```python
from build123d import *

# Parameters (mm, degrees)
F1_DEPTH = 10
F2_DEPTH = 12
F3_SIZE  = 5
F4_SIZE  = 1.99999
F5_R     = 10
F6_DEPTH = 5
F7_R     = 4.99999
F9_DEPTH = 9


# Not quite as in the source:
# - a fillet or chamfer is up to 0.001 mm smaller than in the source, because OpenCascade refuses the exact size


with BuildPart() as f1:
    # F0 (on Right) → F1 (new body)
    with BuildSketch(Plane.YZ):
        with BuildLine():
            Line((15, 5), (27.0370116692, 13))
            ThreePointArc((27.0370116692, 13), (21.2132034356, 21.2132034356), (13, 27.0370116692))
            Line((13, 27.0370116692), (5, 15))
            Line((5, 15), (0, 15))
            Line((0, 15), (-5, 15))
            Line((-5, 15), (-13, 27.0370116692))
            ThreePointArc((-13, 27.0370116692), (-21.2132034356, 21.2132034356), (-27.0370116692, 13))
            Line((-27.0370116692, 13), (-15, 5))
            Line((-15, 5), (-15, 0))
            Line((-15, 0), (-15, -5))
            Line((-15, -5), (-27.0370116692, -13))
            ThreePointArc((-27.0370116692, -13), (-21.2132034356, -21.2132034356), (-13, -27.0370116692))
            Line((-13, -27.0370116692), (-5, -15))
            Line((-5, -15), (0, -15))
            Line((0, -15), (5, -15))
            Line((5, -15), (13, -27.0370116692))
            ThreePointArc((13, -27.0370116692), (21.2132034356, -21.2132034356), (27.0370116692, -13))
            Line((27.0370116692, -13), (15, -5))
            Line((15, -5), (15, 0))
            Line((15, 0), (15, 5))
        make_face()
    extrude(amount=F1_DEPTH)

    # F0 (on Right) → F2 (join)
    with BuildSketch(Plane.YZ):
        with BuildLine():
            ThreePointArc((27.0370116692, -13), (29.2498747867, -6.6666952054), (30, 0))
            ThreePointArc((30, 0), (29.2498747867, 6.6666952054), (27.0370116692, 13))
            Line((27.0370116692, 13), (15, 5))
            Line((15, 5), (15, 0))
            Line((15, 0), (15, -5))
            Line((15, -5), (27.0370116692, -13))
        make_face()
        with BuildLine():
            ThreePointArc((27.0370116692, 13), (29.2498747867, 6.6666952054), (30, 0))
            ThreePointArc((30, 0), (29.2498747867, -6.6666952054), (27.0370116692, -13))
            Line((27.0370116692, -13), (34, -8))
            Line((34, -8), (34, 0))
            Line((34, 0), (34, 8))
            Line((34, 8), (27.0370116692, 13))
        make_face()
        with BuildLine():
            Line((5, 15), (13, 27.0370116692))
            ThreePointArc((13, 27.0370116692), (0, 30), (-13, 27.0370116692))
            Line((-13, 27.0370116692), (-5, 15))
            Line((-5, 15), (0, 15))
            Line((0, 15), (5, 15))
        make_face()
        with BuildLine():
            ThreePointArc((-13, 27.0370116692), (0, 30), (13, 27.0370116692))
            Line((13, 27.0370116692), (8, 34))
            Line((8, 34), (0, 34))
            Line((0, 34), (-8, 34))
            Line((-8, 34), (-13, 27.0370116692))
        make_face()
        with BuildLine():
            Line((-15, 5), (-27.0370116692, 13))
            ThreePointArc((-27.0370116692, 13), (-30, 0), (-27.0370116692, -13))
            Line((-27.0370116692, -13), (-15, -5))
            Line((-15, -5), (-15, 0))
            Line((-15, 0), (-15, 5))
        make_face()
        with BuildLine():
            ThreePointArc((-27.0370116692, -13), (-30, 0), (-27.0370116692, 13))
            Line((-27.0370116692, 13), (-34, 8))
            Line((-34, 8), (-34, 0))
            Line((-34, 0), (-34, -8))
            Line((-34, -8), (-27.0370116692, -13))
        make_face()
        with BuildLine():
            ThreePointArc((-13, -27.0370116692), (0, -30), (13, -27.0370116692))
            Line((13, -27.0370116692), (5, -15))
            Line((5, -15), (0, -15))
            Line((0, -15), (-5, -15))
            Line((-5, -15), (-13, -27.0370116692))
        make_face()
        with BuildLine():
            Line((8, -34), (13, -27.0370116692))
            ThreePointArc((13, -27.0370116692), (0, -30), (-13, -27.0370116692))
            Line((-13, -27.0370116692), (-8, -34))
            Line((-8, -34), (0, -34))
            Line((0, -34), (8, -34))
        make_face()
    extrude(amount=F2_DEPTH)

    # F3
    f3_edges = [f1.edges().sort_by_distance(p)[0] for p in [
        (10, 21.213203, 21.213203),
        (10, -21.213203, 21.213203),
        (10, -21.213203, -21.213203),
        (10, 21.213203, -21.213203),
    ]]
    chamfer(f3_edges, length=F3_SIZE)

    # F4 (size 2 in the source; OpenCascade refuses exactly that, so slightly less here)
    f4_edges = [f1.edges().sort_by_distance(p)[0] for p in [
        (12, 0, 34),
        (12, -10.5, 30.518506),
        (12, 10.5, 30.518506),
        (12, -9, 21.018506),
        (12, 9, 21.018506),
        (12, 0, 15),
        (12, -15, 0),
        (12, -21.018506, 9),
        (12, -30.518506, 10.5),
        (12, -34, 0),
        (12, -30.518506, -10.5),
        (12, -21.018506, -9),
        (12, 0, -15),
        (12, -9, -21.018506),
        (12, -10.5, -30.518506),
        (12, 0, -34),
        (12, 10.5, -30.518506),
        (12, 9, -21.018506),
        (12, 15, 0),
        (12, 21.018506, 9),
        (12, 30.518506, 10.5),
        (12, 34, 0),
        (12, 21.018506, -9),
        (12, 30.518506, -10.5),
    ]]
    chamfer(f4_edges, length=F4_SIZE)

    # F5 (on face) → F6 (join)
    with BuildSketch(Plane.YZ.offset(10)):
        Circle(F5_R)
    extrude(amount=F6_DEPTH)

    # F7 (radius 5 in the source; OpenCascade refuses exactly that, so slightly less here)
    f7_edges = [f1.edges().sort_by_distance(p)[0] for p in [
        (15, -10, 0),
    ]]
    fillet(f7_edges, radius=F7_R)

    # F8 (on face) → F9 (join)
    with BuildSketch(Plane.YZ):
        with BuildLine():
            ThreePointArc((0, -15), (10.6066017178, -10.6066017178), (15, 0))
            ThreePointArc((15, 0), (10.6066017178, 10.6066017178), (0, 15))
            ThreePointArc((0, 15), (-10.6066017178, 10.6066017178), (-15, 0))
            ThreePointArc((-15, 0), (-10.6066017178, -10.6066017178), (0, -15))
        make_face()
    extrude(amount=-F9_DEPTH)


solid = f1.part
```
Could you check a few things on this model? Use its own coordinates, in mm. A direction names the side the tool comes from. Give positions to 0.01 mm unless a question says otherwise; leave off trailing zeros. Write each loop counter-clockwise with the first axis right and the second up, starting at its lowest first coordinate (ties: lowest second). Pieces come first, ordered by that corner, then holes. Notation, with made-up numbers: (-31.75, 57.25) -> (-12.75, 57.25) arc R30 ccw to (-12.75, 89.25) -> close; hole circle Ø10 at (64, 24.25). An arc over 180 degrees is marked (long way). Write each question's results on one line, items separated by ' | '.
1. I want a section at B-B, the plane x = 1.75. Write out the boundary of the cut face in (y, z).
Check sheet entries:
outline: (-34, -8) -> (-27.04, -13) arc R30 ccw to (-13, -27.04) -> (-8, -34) -> (8, -34) -> (13, -27.04) arc R30 ccw to (27.04, -13) -> (34, -8) -> (34, 8) -> (27.04, 13) arc R30 ccw to (13, 27.04) -> (8, 34) -> (-8, 34) -> (-13, 27.04) arc R30 ccw to (-27.04, 13) -> (-34, 8) -> close
2. I need wall thicknesses on L1, parallel to X at y = 26, z = 2; L2, parallel to X at y = 9, z = 0.5; L3, parallel to Y at x = 14, z = -1.5. Which ranges of each line are inside material? Lowest first, please.
Check sheet entries:
L1: x = 0 to 12 | L2: x = -9 to 12.98 | L3: y = -7.86 to 7.86
3. I want a section at D-D, the plane x = 7.5. Write out the boundary of the cut face in (y, z).
Check sheet entries:
outline: (-34, -8) -> (-27.04, -13) -> (-24.93, -11.6) arc R27.5 ccw to (-11.6, -24.93) -> (-13, -27.04) -> (-8, -34) -> (8, -34) -> (13, -27.04) -> (11.6, -24.93) arc R27.5 ccw to (24.93, -11.6) -> (27.04, -13) -> (34, -8) -> (34, 8) -> (27.04, 13) -> (24.93, 11.6) arc R27.5 ccw to (11.6, 24.93) -> (13, 27.04) -> (8, 34) -> (-8, 34) -> (-13, 27.04) -> (-11.6, 24.93) arc R27.5 ccw to (-24.93, 11.6) -> (-27.04, 13) -> (-34, 8) -> close
4. On a 3-axis mill with a long thin cutter (end or side, diameter ignored), from which of +Z, -Z, +X, -X, +Y, -Y can I reach the whole of each face in a straight line? I mean faces 1 (the flat face through (15, 0, 0)), 2 (the flat face through (8.414, 25.449, -11.944)), 3 (the flat face through (8.414, 11.944, 25.449)), 4 (the flat face through (12, -25, 0)). Say none if no direction works.
Check sheet entries:
face 1: +Z, -Z, +X, +Y, -Y | face 2: -Z, +X | face 3: +X, +Y | face 4: +Z, -Z, +X, -Y
5. If we mould it in two halves opening along Y, with no side actions, what happens to faces 5 (the cylindrical face through (2.465, 21.313, 21.113)), 6 (the flat face through (10, 10, -5)), 7 (the flat face through (11.014, -21.664, -8.212)), 8 (the flat face through (10.99, -9.73, -29.89))? For each: released by +Y, released by -Y, zero draft, split by the parting line, or undercut.
Check sheet entries:
face 5: released by +Y | face 6: undercut | face 7: undercut | face 8: released by -Y
6. Will these pins go through, and if not, where does the flat tip stop? pin 1 Ø10 at (x, z) = (-2.5, 20) entering from -Y; pin 2 Ø12 at (y, z) = (3.5, -24.5) entering from +X; pin 3 Ø5 at (y, z) = (-14.5, -5) entering from -X; pin 4 Ø2 at (x, z) = (7, 9.5) entering from +Y.
Check sheet entries:
pin 1: stops at y = -25.58 | pin 2: stops at x = 12 | pin 3: stops at x = -9 | pin 4: stops at y = 33.3
